CAD build for the part. Positions are in the model's coordinates, mm. A direction names the side the tool comes from. Round coordinates to 2 decimals unless told otherwise and drop trailing zeros. Write each loop counter-clockwise with the first axis right and the second up, starting at its lowest first coordinate (ties: lowest second). Pieces come first, ordered by that corner, then holes. Notation, with made-up numbers: (-7, 68.5) - (32, 68.5) arc R23 ccw to (32, 77.5) - close; hole circle Ø3 at (-4.5, 46). An arc over 180 degrees is marked (long way). Answer in a Markdown table with one row per item.
Autodesk Inventor part; units mm, degrees
ref_plane "YZ Plane" through (0, 0, 0) normal (1, 0, 0) x (0, 1, 0)
ref_plane "XZ Plane" through (0, 0, 0) normal (0, 1, 0) x (-1, 0, 0)
ref_plane "XY Plane" through (0, 0, 0) normal (0, 0, 1) x (1, 0, 0)
sketch "Sketch1" plane through (0, 0, 0) normal (0, 0, 1) x (1, 0, 0)
  circle A0 centre (0, 0) radius 68.75
  circle A1 centre (0, 0) radius 15
  circle A2 centre (-40, 0) radius 4
  line L0 (-49, 9) -> (-31, 9) construction
  line L1 (-31, 9) -> (-31, -9) construction
  line L2 (-31, -9) -> (-49, -9) construction
  line L3 (-49, -9) -> (-49, 9) construction
  circle A3 centre (-49, 9) radius 2
  circle A4 centre (-31, 9) radius 2
  circle A5 centre (-31, -9) radius 2
  circle A6 centre (-49, -9) radius 2
  circle A7 centre (20, 34.641) radius 3.5
  line L4 (0, 0) -> (-40, 0) construction
  line L5 (0, 0) -> (20, 34.641) construction
  line L6 (0, 0) -> (20, -34.641) construction
  circle A8 centre (20, -34.641) radius 3.5
  point P0 (-49, 0)
  point P1 (-40, 9)
  dimension "d0" = 137.5
  dimension "d1" = 30
  dimension "d2" = 8
  dimension "d3" = 40
  dimension "d4" = 18
  dimension "d5" = 18
  dimension "d6" = 4
  dimension "d7" = 4
  dimension "d8" = 4
  dimension "d9" = 4
  dimension "d10" = 7
  dimension "d11" = 40
  dimension "d12" = 120
  dimension "d13" = 40
  dimension "d14" = 7
  dimension "d15" = 120
extrude "Extrusion1" add sketch "Sketch1" along normal blind 5
sketch "Sketch2" plane through (0, 0, 5) normal (0, 0, 1) x (1, 0, 0)
  circle A0 centre (0, 0) radius 68.75
  circle A1 centre (0, 0) radius 63.75
  dimension "d18" = 5
extrude "Extrusion2" add sketch "Sketch2" along normal blind 115
sketch "Sketch3" plane through (0, 0, 5) normal (0, 0, 1) x (1, 0, 0)
  circle A0 centre (-40, 0) radius 4
  circle A1 centre (0, 0) radius 15
  circle A2 centre (20, 34.641) radius 3.5
  circle A3 centre (20, -34.641) radius 3.5
  circle A4 centre (-40, 0) radius 20
  line L0 (26.8253, 21.4628) -> (5.1747, 33.9628)
  line L1 (5.1747, 33.9628) -> (13.1747, 47.8192)
  line L2 (13.1747, 47.8192) -> (34.8253, 35.3192)
  line L3 (34.8253, 35.3192) -> (26.8253, 21.4628)
  line L4 (26.8253, 21.4628) -> (13.1747, 47.8192) construction
  line L5 (5.1747, 33.9628) -> (34.8253, 35.3192) construction
  line L6 (0, 0) -> (-40, 0) construction
  line L7 (5.1747, -33.9628) -> (26.8253, -21.4628)
  line L8 (26.8253, -21.4628) -> (34.8253, -35.3192)
  line L9 (34.8253, -35.3192) -> (13.1747, -47.8192)
  line L10 (13.1747, -47.8192) -> (5.1747, -33.9628)
  circle A5 centre (0, 0) radius 63.75
  dimension "d21" = 40
  dimension "d23" = 120
  dimension "d24" = 16
  dimension "d25" = 25
  dimension "d28" = 120
extrude "Extrusion3" add sketch "Sketch3" along normal blind 100 contours A5
sketch "Sketch4" plane through (0, 0, 105) normal (0, 0, 1) x (1, 0, 0)
  circle A0 centre (50, 0) radius 3
  circle A1 centre (-25, 43.3013) radius 3
  circle A2 centre (-25, -43.3013) radius 3
  circle A3 centre (50, 0) radius 15
  circle A4 centre (-25, 43.3013) radius 15
  circle A5 centre (-25, -43.3013) radius 15
  point P0 (0, 0)
  dimension "d32" = 6
  dimension "d33" = 50
  dimension "d36" = 360
  dimension "d38" = 30
  dimension "d39" = 30
  dimension "d40" = 30
extrude "Extrusion4" add sketch "Sketch4" along normal blind 15
sketch "Sketch6" plane through (-40, 0, 5) normal (0, 0, 1) x (1, 0, 0)
  circle A0 centre (0, 0) radius 4
  circle A1 centre (0, 0) radius 16.5
  circle A2 centre (0, 0) radius 20
  point P0 (40, 0)
  point P1 (20, 0)
  dimension "d46" = 33
extrude "Extrusion6" add sketch "Sketch6" along normal blind 40 contours A2
sketch "Sketch7" plane through (0, 0, 120) normal (0, 0, 1) x (1, 0, 0)
  circle A0 centre (37, 64.0859) radius 10
  line L0 (28.3397, 69.0859) -> (25.3492, 63.906)
  line L1 (45.6603, 59.0859) -> (42.6697, 53.906)
  circle A1 centre (0, 0) radius 68.75 construction
  line L2 (0, 0) -> (37, 64.0859) construction
  line L3 (25.3492, 63.906) -> (42.6697, 53.906)
  circle A2 centre (20, 34.641) radius 3.5
  circle A3 centre (37, 64.0859) radius 3
  circle A4 centre (-37, 64.0859) radius 10
  line L4 (-45.6603, 59.0859) -> (-42.6697, 53.906)
  line L5 (-28.3397, 69.0859) -> (-25.3492, 63.906)
  line L6 (-42.6697, 53.906) -> (-25.3492, 63.906)
  circle A5 centre (-37, 64.0859) radius 3
  circle A6 centre (-74, 0) radius 10
  line L7 (-74, -10) -> (-68.0188, -10)
  line L8 (-74, 10) -> (-68.0188, 10)
  line L9 (-68.0188, -10) -> (-68.0188, 10)
  circle A7 centre (-74, 0) radius 3
  circle A8 centre (-37, -64.0859) radius 10
  line L10 (-28.3397, -69.0859) -> (-25.3492, -63.906)
  line L11 (-45.6603, -59.0859) -> (-42.6697, -53.906)
  line L12 (-25.3492, -63.906) -> (-42.6697, -53.906)
  circle A9 centre (-37, -64.0859) radius 3
  circle A10 centre (37, -64.0859) radius 10
  line L13 (45.6603, -59.0859) -> (42.6697, -53.906)
  line L14 (28.3397, -69.0859) -> (25.3492, -63.906)
  line L15 (42.6697, -53.906) -> (25.3492, -63.906)
  circle A11 centre (37, -64.0859) radius 3
  circle A12 centre (74, 0) radius 10
  line L16 (74, 10) -> (68.0188, 10)
  line L17 (74, -10) -> (68.0188, -10)
  line L18 (68.0188, 10) -> (68.0188, -10)
  circle A13 centre (74, 0) radius 3
  dimension "d49" = 20
  dimension "d52" = 74
  dimension "d53" = 6
  dimension "d56" = 360
extrude "Extrusion7" add sketch "Sketch7" against normal blind 20 contours A0 L3 | A0 L3 L0 | L1 L3 A0 | L3 A0 | A4 L6 | A4 L5 L6 | A4 L6 | A4 L6 L4 | A6 L9 | L8 L9 A6 | A6 L9 L7 | A6 L9 | A8 L12 | L11 L12 A8 | A8 L12 L10 | A8 L12 | A10 L15 | A10 L15 L13 | L14 L15 A10 | L15 A10 | A12 L18 | A12 L18 L16 | L17 L18 A12 | L18 A12
sketch "Sketch8" plane through (0, 0, 105) normal (0, 0, 1) x (1, 0, 0)
  circle A0 centre (0, 0) radius 63.75
  dimension "d62" = 127.5
extrude "Extrusion8" cut sketch "Sketch8" along normal through all
properties part number "TA02" material "ABS Plastic"
Q1. Saw through at D-D on z = 113.5. Count the separate pieces of the cut face and the enclosed holes in it, then the cut area to 3 significant figures.
Computed:
| item | result |
|---|---|
| separate pieces | 1 |
| enclosed holes | 7 |
| area | 3,510 mm2 |
Q2. Saw through at B-B on x = 0. List the corners of the cut face in (y, z), then the cut area to 3 significant figures.
Computed:
| item | result |
|---|---|
| outline | (-68.75, 0) - (-15, 0) - (-15, 105) - (-63.75, 105) - (-63.75, 120) - (-68.75, 120) - close; (15, 0) - (68.75, 0) - (68.75, 120) - (63.75, 120) - (63.75, 105) - (15, 105) - close |
| area | 11,400 mm2 |
Q3. Drill centre lines: line 1 (Y direction, x = -31, z = 1); line 2 (Y direction, x = -74, z = 106); line 3 (Y direction, x = 37, z = 112). Where is each one in solid material? Low to high.
Computed:
| item | result |
|---|---|
| line 1 | y = -61.36 to -11, -7 to 7, 11 to 61.36 |
| line 2 | y = -10 to -3, 3 to 10 |
| line 3 | y = -74.09 to -67.09, -61.09 to -51.91, 51.91 to 61.09, 67.09 to 74.09 |
Q4. Flat gauge pins, fed straight in: pin 1 (1.5 mm diameter, centred on y = 12.5, z = 23, fed in from -X); pin 2 (6 mm diameter, centred on y = 6.5, z = 29, fed in from -X); pin 3 (5 mm diameter, centred on x = -79.5, y = 1.5, fed in from -Z). Where does each tip first touch, or does it go through?
Computed:
| item | result |
|---|---|
| pin 1 | stops at x = -67.74 |
| pin 2 | stops at x = -68.66 |
| pin 3 | stops at z = 100 |
Q5. Saw through at A-A on z = 95. List the corners of the cut face in (x, y), then the cut area to 3 significant figures.
Computed:
| item | result |
|---|---|
| outline | circle Ø137.5 at (0, 0); hole circle Ø40 at (-40, 0); hole circle Ø30 at (0, 0); hole (5.17, -33.96) - (13.17, -47.82) - (34.83, -35.32) - (26.83, -21.46) - close; hole (5.17, 33.96) - (26.83, 21.46) - (34.83, 35.32) - (13.17, 47.82) - close |
| area | 12,100 mm2 |
Q6. 3-axis set-ups, long thin cutter, end or side, ignore diameter. For faces 4 (the flat face through (16, 35, 5)), 5 (the flat face through (71, -10, 110)), 6 (the flat face through (38, -68, 100)), 7 (the flat face through (71, 10, 110)), 8 (the flat face through (-71, 10, 110)): which of +Z, -Z, +X, -X, +Y, -Y reach the whole face in a straight line?
Computed:
| item | result |
|---|---|
| face 4 | +Z |
| face 5 | +Z, -Z, +X, -Y |
| face 6 | -Z, +X, -Y |
| face 7 | +Z, -Z, +X, +Y |
| face 8 | +Z, -Z, -X, +Y |
Q7. Saw through at C-C on x = 20. List the corners of the cut face in (y, z), then the cut area to 3 significant figures.
Computed:
| item | result |
|---|---|
| outline | (-65.78, 0) - (-38.14, 0) - (-38.14, 5) - (-43.88, 5) - (-43.88, 105) - (-60.53, 105) - (-60.53, 120) - (-65.78, 120) - close; (-31.14, 0) - (31.14, 0) - (31.14, 5) - (25.4, 5) - (25.4, 105) - (-25.4, 105) - (-25.4, 5) - (-31.14, 5) - close; (38.14, 0) - (65.78, 0) - (65.78, 120) - (60.53, 120) - (60.53, 105) - (43.88, 105) - (43.88, 5) - (38.14, 5) - close |
| area | 10,200 mm2 |
Q8. Pull direction X, two halves, no side cores. Call faces 1 (the flat face through (62, 17, 120)), 2 (the cylindrical face through (-84, 0, 110)), 3 (the flat face through (9.119, 40.794, 54.3)): released by +X, released by -X, zero draft, split by the parting line, or undercut.
Computed:
| item | result |
|---|---|
| face 1 | zero draft |
| face 2 | released by -X |
| face 3 | undercut |
